Here's how the part is built. I have some questions about the finished solid (model axes, mm). Face numbers are marked on the shaded views. A direction names the side the tool comes from. Round coordinates to 2 decimals unless told otherwise and drop trailing zeros. Order: outer loops, then holes, each group sorted by start corner. A loop starts at its lowest first (then second) coordinate and runs counter-clockwise, first axis right, second up. Notation, with made-up numbers: (32.25, 53) - (60.25, 53) arc R12 ccw to (60.25, 67) - close; hole circle Ø1 at (-19, 33.5). An arc over 180 degrees is marked (long way). One line per item, written item: value.
Solid Edge part; units mm, degrees
sketch "Sketch1" plane through (0, 0, 0) normal (0, 0, 1) x (1, 0, 0)
  line L0 (30, 40) -> (30, 0)
  line L1 (0, 0) -> (30, 0)
  line L2 (0, 0) -> (-30, 0)
  line L3 (-30, 0) -> (-30, 40)
  line L4 (-30, 40) -> (30, 40)
extrude "Protrusion1" add sketch "Sketch1" against normal blind 20
sketch "Sketch2" plane through (0, 0, 0) normal (0, 0, 1) x (1, 0, 0)
  circle A0 centre (0, 40) radius 30
extrude "ExtrudedProtrusion_2" add sketch "Sketch2" against normal blind 20 and the other way blind 40
sketch "Sketch3" plane through (0, 0, 0) normal (0, 0, 1) x (1, 0, 0)
  line L0 (-30, 20) -> (30, 20)
  line L1 (30, 20) -> (30, 0)
  line L2 (30, 0) -> (-30, 0)
  line L3 (-30, 0) -> (-30, 20)
extrude "ExtrudedProtrusion_4" add sketch "Sketch3" against normal blind 60
sketch "Sketch4" plane through (0, 0, 0) normal (1, 0, 0) x (0, 1, 0)
  circle A0 centre (0, -66) radius 30
extrude "ExtrudedProtrusion_5" add sketch "Sketch4" along normal mid plane 80
sketch "Sketch5" plane through (0, 0, 0) normal (1, 0, 0) x (0, 1, 0)
  circle A0 centre (0, -66) radius 15
extrude "ExtrudedCutout_1" cut sketch "Sketch5" along normal mid plane 80
sketch "Sketch6" plane through (0, 0, 0) normal (1, 0, 0) x (0, 1, 0)
  line L0 (0, 0) -> (-26.7217, -52.3636)
  line L1 (0, -36) -> (0, 0)
  arc A0 (-26.7217, -52.3636) -> (0, -36) centre (0, -66) cw
extrude "ExtrudedProtrusion_6" add sketch "Sketch6" along normal mid plane 12
sketch "Sketch7" plane through (0, 40, 40) normal (0, 0, 1) x (0, 1, 0)
  circle A0 centre (0, 0) radius 10
extrude "Cutout1" cut sketch "Sketch7" against normal up to vertex (40 mm away)
sketch "Sketch8" plane through (0, 0, 0) normal (1, 0, 0) x (0, 1, 0)
  line L0 (10, 40) -> (10, 0)
  line L1 (10, 0) -> (20, 40)
  line L2 (20, 40) -> (10, 40)
revolve "RevolvedCutout_2" cut sketch "Sketch8" angle 350.433 about axis through (0, 40, 40) along (0, 0, 1)
sketch "Sketch9" plane through (0, 0, 0) normal (1, 0, 0) x (0, 1, 0)
  line L0 (20, 40) -> (10, 40)
  line L1 (10, 40) -> (10, 0)
  line L2 (10, 0) -> (20, 40)
extrude "ExtrudedCutout_3" cut sketch "Sketch9" against normal blind 14.7249
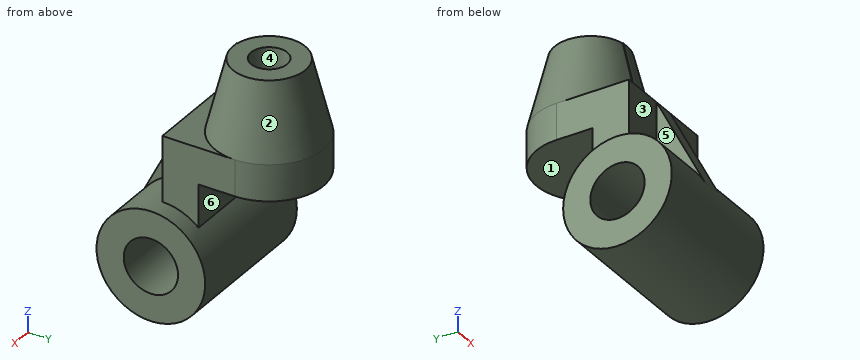
Q1. If I drill on line 1 along Y through (x, z) = (15.5, -65); line 2 along Z through (x, y) = (5, 0); line 3 along X through (y, z) = (6, -14.5), over which ranges is the centre line in solid material (lowest first)?
Results list:
line 1: -29.98 to -14.97, 14.97 to 29.98
line 2: -96 to -81, -51 to 0
line 3: -30 to 30
Q2. Which directions (+Z, -Z, +X, -X, +Y, -Y) give clear straight access to the entire face, cutting with the end or side of a thin tool? Please do the marked faces 4, 5 and 6.
Results list:
face 4: +Z
face 5: +Z, -X, -Y
face 6: +X, -X, +Y
Q3. We'd pull the mould along Z, two halves only. Please class the marked faces 1, 2 and 3: released by +Z, released by -Z, zero draft, split by the parting line, or undercut.
Results list:
face 1: undercut
face 2: released by +Z
face 3: zero draft
Q4. Will these pins go through, and if not, where does the flat tip stop? pin 1 (12 mm diameter, centred on x = 17, z = -70, fed in from +Y); pin 2 (16 mm diameter, centred on x = 0, y = 40, fed in from -Z); pin 3 (5 mm diameter, centred on x = -12, y = 14.5, fed in from -Z).
Results list:
pin 1: y = 30
pin 2: z = -20
pin 3: z = -93.5
Q5. If we section it at D-D, the plane y = -20.5: Please give me the cut outline in (x, z), then the cut area to 3 significant figures.
Results list:
outline: (-40, -87.9) - (40, -87.9) - (40, -44.1) - (6, -44.1) - (6, -40.17) - (-6, -40.17) - (-6, -44.1) - (-40, -44.1) - close
area: 3,550 mm²
Q6. If we section it at B-B, the plane y = 5: Please give me the cut outline in (x, z), then the cut area to 3 significant figures.
Results list:
outline: (-40, -95.58) - (40, -95.58) - (40, -80.14) - (-40, -80.14) - close; (-40, -51.86) - (40, -51.86) - (40, -36.42) - (30, -36.42) - (30, 0) - (-30, 0) - (-30, -36.42) - (-40, -36.42) - close
area: 4,660 mm²
Q7. If we section it at C-C, the plane z = -27: Please give me the cut outline in (x, y).
Results list:
outline: (-30, 0) - (-6, 0) - (-6, -13.78) - (6, -13.78) - (6, 0) - (30, 0) - (30, 20) - (-30, 20) - close
Q8. If we section it at A-A, the plane z = -66: Please give me the cut outline in (x, y).
Results list:
outline: (-40, -30) - (40, -30) - (40, -15) - (-40, -15) - close; (-40, 15) - (40, 15) - (40, 30) - (-40, 30) - close
